```python
from build123d import *

# Parameters (mm, degrees)
F0_R     = 3
F0_W     = 9
F0_H     = 6
F0_W_2   = 4
F0_W_3   = 13.5
F1_DEPTH = 10.5
F2_DEPTH = 4
F3_R     = 2


with BuildPart() as f1:
    # F0 (on Top) → F1 (new body)
    with BuildSketch(Plane.XY):
        Polygon((27.5, 10), (-27.5, 10), (-27.5, -10), (27.5, -10), (27.5, -3), (14, -3), (14, 3), (27.5, 3), align=None)
        with Locations((-19, 0)):
            Circle(F0_R, mode=Mode.SUBTRACT)
        with Locations((-6.5, 0)):
            Rectangle(F0_W, F0_H, mode=Mode.SUBTRACT)
        with Locations((6, 0)):
            Circle(F0_R, mode=Mode.SUBTRACT)
        with Locations((29.5, 0)):
            Rectangle(F0_W_2, F0_H)
        with Locations((20.75, 0)):
            Rectangle(F0_W_3, F0_H)
        with Locations((-6.5, 0)):
            Rectangle(F0_W, F0_H)
    extrude(amount=-F1_DEPTH)

    # F0 (on Top) → F2 (join)
    with BuildSketch(Plane.XY):
        with Locations((20.75, 0)):
            Rectangle(F0_W_3, F0_H)
        with Locations((29.5, 0)):
            Rectangle(F0_W_2, F0_H)
        with Locations((-6.5, 0)):
            Rectangle(F0_W, F0_H)
    extrude(amount=F2_DEPTH)

    # F3
    f3_edges = [f1.edges().sort_by_distance(p)[0] for p in [
        (22.75, -3, 4),
        (22.75, 3, 4),
        (31.5, 3, -3.25),
        (31.5, -3, -3.25),
        (-6.5, 3, 4),
        (-6.5, -3, 4),
    ]]
    fillet(f3_edges, radius=F3_R)


solid = f1.part
```
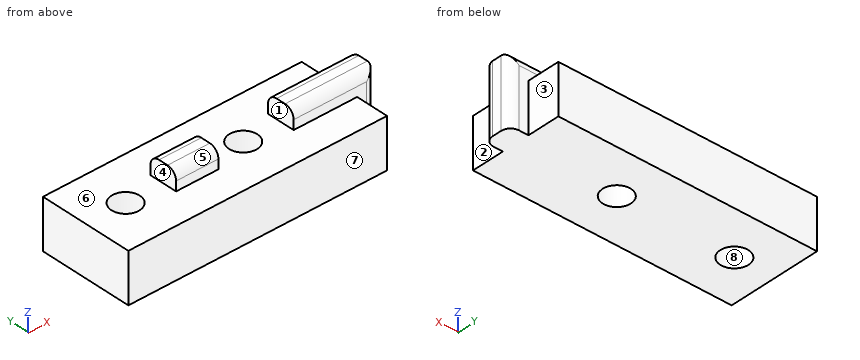
Can you work these out from the model? Positions are in its coordinate system, mm. Face numbers are marked on the shaded views. A direction names the side the tool comes from. Coordinates: 2 decimals unless noted, no trailing zeros. Order: outer loops, then holes, each group sorted by start corner. A loop starts at its lowest first (then second) coordinate and runs counter-clockwise, first axis right, second up.
1. If we section it at B-B (z = -6): Please give me the cut outline in (x, y).
2. If we section it at D-D (x = 15.5): Please give me the cut outline in (y, z), then the cut area to 3 significant figures.
3. For the marked faces 1, 2, 3, 4 and 5, which set-ups out of +Z, -Z, +X, -X, +Y, -Y let a thin tool reach every point of the face, with its end or its side?
4. I'm going to push flat-ended pins straight in: pin 1 (4 mm diameter, centred on x = -17.5, y = 5.5, fed in from +Z); pin 2 (3.5 mm diameter, centred on y = 8, z = -7, fed in from +X); pin 3 (7.5 mm diameter, centred on y = -6, z = -7, fed in from +X). Where does each tip first touch, or does it pass through?
5. I need wall thicknesses on line 1 (Y direction, x = -19, z = -6.75); line 2 (X direction, y = -0.75, z = -5.75); line 3 (X direction, y = -1, z = 3.25). Which ranges of each line are inside material? Lowest first, please.
6. If we section it at A-A (x = -19): Please give me the cut outline in (y, z).
7. Thinking about a two-plate mould opening in Y: for the marked faces 6, 7 and 8, which applies, +Y half, -Y half, draft (parallel to the pull), parting line (faces both ways), or undercut?
8. If we section it at C-C (y = 1.75): Please give me the cut outline in (x, z).
Entries:
1. outline: (-27.5, -10) - (27.5, -10) - (27.5, -3) - (29.5, -3) arc R2 ccw to (31.5, -1) - (31.5, 1) arc R2 ccw to (29.5, 3) - (27.5, 3) - (27.5, 10) - (-27.5, 10) - close; hole circle Ø6 at (-19, 0); hole circle Ø6 at (6, 0)
2. outline: (-10, -10.5) - (10, -10.5) - (10, 0) - (3, 0) - (3, 2) arc R2 ccw to (1, 4) - (-1, 4) arc R2 ccw to (-3, 2) - (-3, 0) - (-10, 0) - close
2. area: 232 mm2
3. face 1: +Z, +Y, -Y
3. face 2: +Z, -Z, +X, -Y
3. face 3: +Z, -Z, +X, +Y
3. face 4: +Z, -X, +Y, -Y
3. face 5: +Z, +X, -X, -Y
4. pin 1: stops at z = 0
4. pin 2: stops at x = 27.5
4. pin 3: stops at x = 31.06
5. line 1: y = -10 to -3, 3 to 10
5. line 2: x = -27.5 to -21.9, -16.1 to 3.1, 8.9 to 31.5
5. line 3: x = -11 to -2, 14 to 31.5
6. outline: (-10, -10.5) - (-3, -10.5) - (-3, 0) - (-10, 0) - close; (3, -10.5) - (10, -10.5) - (10, 0) - (3, 0) - close
7. face 6: draft
7. face 7: -Y half
7. face 8: undercut
8. outline: (-27.5, -10.5) - (-21.44, -10.5) - (-21.44, 0) - (-27.5, 0) - close; (-16.56, -10.5) - (3.56, -10.5) - (3.56, 0) - (-2, 0) - (-2, 3.85) - (-11, 3.85) - (-11, 0) - (-16.56, 0) - close; (8.44, -10.5) - (31.35, -10.5) - (31.35, 3.85) - (14, 3.85) - (14, 0) - (8.44, 0) - close
